```python
from build123d import *

# Parameters (mm, degrees)
F2_R     = 12.7
F3_DEPTH = 101.6


with BuildPart() as f1:
    # F0 (on Top) → F1 (revolve)
    with BuildSketch(Plane.XY):
        with BuildLine():
            Line((0, 0), (0, -38.1))
            ThreePointArc((0, -38.1), (38.1, 0), (0, 38.1))
            Line((0, 38.1), (0, 0))
        make_face()
    revolve(axis=Axis((0, 0, 0), (0, 1, 0)))

    # F2 (on Front) → F3 (join)
    with BuildSketch(Plane.XZ):
        Circle(F2_R)
    extrude(amount=F3_DEPTH)

    # F5 (on offset) → F6 (revolve)
    with BuildSketch(Plane.XZ.offset(107.95)):
        with BuildLine():
            Line((0, 0), (-25.4, 0))
            ThreePointArc((-25.4, 0), (0, -25.4), (25.4, 0))
            Line((25.4, 0), (0, 0))
        make_face()
    revolve(axis=Axis((0, -107.95, 0), (1, 0, 0)))


solid = f1.part
```
Source: CAD feature listing. Evaluate the final solid. Frame: model axes, mm. Round coordinates to 2 decimals unless told otherwise and drop trailing zeros. Write each loop counter-clockwise with the first axis right and the second up, starting at its lowest first coordinate (ties: lowest second). Pieces come first, ordered by that corner, then holes. Notation, with made-up numbers: M -6,19.5 L 27,19.5 A10 cw 27,38.5 Z; hole C 83.25,-8 d6. An arc over 180 degrees is marked long. Answer as a JSON object with one key per item and string values. Group by question number.
(1) Section query D-D on z = -23.5. Output: boundary loops of the cut face in (x, y).
(2) Section query A-A on z = 0. Output: boundary loops of the cut face in (x, y), then the cut area to 3 significant figures.
(3) Section query B-B on x = 17. Output: boundary loops of the cut face in (y, z).
(4) Section query C-C on x = 0. Output: boundary loops of the cut face in (y, z), then the cut area to 3 significant figures.
(5) Ray query, line 1 (Y direction, x = -14, z = 18); line 2 (Y direction, x = 16.5, z = 31); line 3 (Y direction, x = -19, z = 28.5). Return the intervals inside material, ascending. Write a range as [from, to].
(6) First-contact query: pin 1 (4 mm diameter, centred on y = -80, z = -1.5, fed in from +X); pin 2 (12 mm diameter, centred on x = 15.5, z = -27.5, fed in from -Y); pin 3 (6 mm diameter, centred on y = -10.5, z = 29.5, fed in from +X). Flat tips, straight axial feed; report the tip coordinate or a pass-through.
Computed values:
{
 "1": {"outline": "C 0,0 d59.98; C 0,-107.95 d19.28"},
 "2": {"outline": "M -12.7,-85.95 A25.4 ccw long 12.7,-85.95 L 12.7,-35.92 A38.1 ccw long -12.7,-35.92 Z", "area": "7,760 mm^2"},
 "3": {"outline": "C -107.95,0 d37.74; C 0,0 d68.19"},
 "4": {"outline": "M -85.95,-12.7 L -35.92,-12.7 A38.1 ccw long -35.92,12.7 L -85.95,12.7 A25.4 ccw long Z", "area": "7,760 mm^2"},
 "5": {"line 1": "[-119.14, -96.76], [-30.52, 30.52]", "line 2": "[-14.78, 14.78]", "line 3": "[-16.68, 16.68]"},
 "6": {"pin 1": "x = 12.7", "pin 2": "y = -28.25", "pin 3": "x = 25.49"}
}
